CAD build for the part. Positions are in the model's coordinates, mm. A direction names the side the tool comes from. Round coordinates to 2 decimals unless told otherwise and drop trailing zeros. Loops run counter-clockwise (first coordinate to the right, second up) from the corner with the lowest first, then second, coordinate; pieces in that order, holes last. Notation, with made-up numbers: M 57,34.5 L 109,34.5 A20 ccw 109,50.5 Z; hole C 25,-21.75 d4. An arc over 180 degrees is marked long. One line per item, written item: value. Start each with the question number.
from build123d import *

# Parameters (mm, degrees)
SKETCH1_W           = 105
SKETCH1_H           = 70
BOSS_EXTRUDE1_DEPTH = 15
SKETCH3_W           = 98
SKETCH3_H           = 63
CUT_EXTRUDE1_DEPTH  = 12
FILLET1_R           = 6
SKETCH4_R           = 3.5
BOSS_EXTRUDE2_DEPTH = 5
SKETCH5_R           = 1
CUT_EXTRUDE2_DEPTH  = 8
SKETCH6_W           = 3.5
SKETCH6_H           = 18.3
SKETCH6_W_2         = 14
SKETCH6_H_2         = 3.5
SKETCH6_H_3         = 20
CUT_EXTRUDE3_DEPTH  = 6
BOSS_EXTRUDE3_DEPTH = 3
FILLET2_R           = 0.5


with BuildPart() as part:
    # Sketch1 → Boss-Extrude1 (new body)
    with BuildSketch(Plane(origin=(0, 0, 0), x_dir=(1, 0, 0), z_dir=(0, 1, 0))):
        Rectangle(SKETCH1_W, SKETCH1_H)
    extrude(amount=BOSS_EXTRUDE1_DEPTH)

    # Sketch3 → Cut-Extrude1 (cut)
    with BuildSketch(Plane(origin=(0, 15, 0), x_dir=(1, 0, 0), z_dir=(0, 1, 0))):
        Rectangle(SKETCH3_W, SKETCH3_H)
    extrude(amount=-CUT_EXTRUDE1_DEPTH, mode=Mode.SUBTRACT)

    # Fillet1
    fillet1_edges = [part.edges().sort_by_distance(p)[0] for p in [
        (-49, 9, 31.5),
        (-49, 9, -31.5),
        (49, 9, -31.5),
        (49, 9, 31.5),
        (52.5, 7.5, 35),
        (-52.5, 7.5, 35),
        (-52.5, 7.5, -35),
        (52.5, 7.5, -35),
    ]]
    fillet(fillet1_edges, radius=FILLET1_R)

    # Sketch4 → Boss-Extrude2 (add)
    with BuildSketch(Plane(origin=(0, 3, 0), x_dir=(1, 0, 0), z_dir=(0, 1, 0))):
        with Locations(Location((40, -22.5, 0), (0, 0, 270))):
            Circle(SKETCH4_R)
        with Locations(Location((40, 19.2, 0), (0, 0, 270))):
            Circle(SKETCH4_R)
        with Locations(Location((-36.1, -22.5, 0), (0, 0, 270))):
            Circle(SKETCH4_R)
        with Locations(Location((-36.1, 19.2, 0), (0, 0, 270))):
            Circle(SKETCH4_R)
    extrude(amount=BOSS_EXTRUDE2_DEPTH)

    # Sketch5 → Cut-Extrude2 (cut)
    with BuildSketch(Plane(origin=(0, 8, 0), x_dir=(1, 0, 0), z_dir=(0, 1, 0))):
        with Locations(Location((-36.1, 19.2, 0), (0, 0, 270))):
            Circle(SKETCH5_R)
        with Locations(Location((-36.1, -22.5, 0), (0, 0, 270))):
            Circle(SKETCH5_R)
        with Locations(Location((40, -22.5, 0), (0, 0, 270))):
            Circle(SKETCH5_R)
        with Locations(Location((40, 19.06026255, 0), (0, 0, 270))):
            Circle(SKETCH5_R)
    extrude(amount=-CUT_EXTRUDE2_DEPTH, mode=Mode.SUBTRACT)

    # Sketch6 → Cut-Extrude3 (cut)
    with BuildSketch(Plane(origin=(0, 15, 0), x_dir=(1, 0, 0), z_dir=(0, 1, 0))):
        with Locations((50.75, 0.51)):
            Rectangle(SKETCH6_W, SKETCH6_H)
        with Locations((27.76, -33.25)):
            Rectangle(SKETCH6_W_2, SKETCH6_H_2)
        with Locations((-50.75, 0)):
            Rectangle(SKETCH6_W, SKETCH6_H_3)
    extrude(amount=-CUT_EXTRUDE3_DEPTH, mode=Mode.SUBTRACT)

    # Sketch7 → Boss-Extrude3 (add)
    with BuildSketch(Plane(origin=(0, 15, 0), x_dir=(1, 0, 0), z_dir=(0, 1, 0))):
        with BuildLine():
            Line((-44.5, 33), (44.5, 33))
            ThreePointArc((44.5, 33), (48.742640687, 31.242640687), (50.5, 27))
            Line((50.5, 27), (50.5, 9.736559035))
            Line((50.5, 9.736559035), (48.5, 9.736559035))
            Line((48.5, 9.736559035), (48.5, 25))
            ThreePointArc((48.5, 25), (46.742640687, 29.242640687), (42.5, 31))
            Line((42.5, 31), (-42.5, 31))
            ThreePointArc((-42.5, 31), (-46.742640687, 29.242640687), (-48.5, 25))
            Line((-48.5, 25), (-48.5, 10))
            Line((-48.5, 10), (-50.5, 10))
            Line((-50.5, 10), (-50.5, 27))
            ThreePointArc((-50.5, 27), (-48.742640687, 31.242640687), (-44.5, 33))
        make_face()
        with BuildLine():
            Line((-44.5, -33), (20.754470261, -33))
            Line((20.754470261, -33), (20.754470261, -31))
            Line((20.754470261, -31), (-42.5, -31))
            ThreePointArc((-42.5, -31), (-46.742640687, -29.242640687), (-48.5, -25))
            Line((-48.5, -25), (-48.5, -10.02702289))
            Line((-48.5, -10.02702289), (-50.5, -10.02702289))
            Line((-50.5, -10.02702289), (-50.5, -27))
            ThreePointArc((-50.5, -27), (-48.742640687, -31.242640687), (-44.5, -33))
        make_face()
        with BuildLine():
            Line((50.5, -8.739580153), (50.5, -27))
            ThreePointArc((50.5, -27), (48.742640687, -31.242640687), (44.5, -33))
            Line((44.5, -33), (34.809182833, -33))
            Line((34.809182833, -33), (34.809182833, -31))
            Line((34.809182833, -31), (42.5, -31))
            ThreePointArc((42.5, -31), (46.742640687, -29.242640687), (48.5, -25))
            Line((48.5, -25), (48.5, -8.739580153))
            Line((48.5, -8.739580153), (50.5, -8.739580153))
        make_face()
    extrude(amount=BOSS_EXTRUDE3_DEPTH)

    # Fillet2
    fillet2_edges = [part.edges().sort_by_distance(p)[0] for p in [
        (49, 15, 17.119790077),
        (47.242640687, 15, 29.742640687),
        (-49, 15, 17.763511445),
        (-47.242640687, 15, 29.742640687),
        (49, 15, -17.618279517),
        (47.242640687, 15, -29.742640687),
        (-49, 15, -17.75),
        (-47.242640687, 15, -29.742640687),
        (38.904591417, 15, 31.5),
        (-11.12276487, 15, 31.5),
        (0, 15, -31.5),
    ]]
    fillet(fillet2_edges, radius=FILLET2_R - 0.0001)  # a hair under: the kernel refuses the full size


solid = part.part
(1) Flat gauge pins, fed straight in: P1, Ø0.6, axis at y = 17, z = 32, coming from the -X side; P2, Ø7.5, axis at x = -37, z = -20.5, coming from the +Y side; P3, Ø3, axis at y = 12.5, z = 32.5, coming from the +X side; P4, Ø4, axis at x = 28.5, y = 9.5, coming from the +Z side. Where does each tip first touch, or does it go through?
(2) Slice it at A-A, the plane y = 13.25. List the corners of the cut face in (x, z), and give its area (3 significant figures).
(3) Probe L1, parallel to X at y = 3.25, z = 22.5; L2, parallel to X at y = 6.75, z = 24; L3, parallel to Z at x = -6, y = 9.5. List the from-to ranges inside material, lowest first.
(4) Slice it at D-D, the plane z = 3.5. List the corners of the cut face in (x, y).
(5) Which spindle directions (+Z, -Z, +X, -X, +Y, -Y) get a long thin tool onto all of the face, cutting with end or side? Do faces 4 (the flat face through (-50.5, 16, -18)), 5 (the cylindrical face through (-32.63, 5.46, 22.04)), 6 (the flat face through (34.809, 17, 32)), 7 (the flat face through (-49, 17, 10.027)). Say none if no direction does.
(6) Mould opens along X. For faces 1 (the cylindrical face through (-35.26, 4.06, 23.04)), 2 (the flat face through (11, 18, -32)), 3 (the cylindrical face through (48.789, 16.479, 31.196)) say: pulls with the +X half, pulls with the -X half, needs draft (parallel to the pull), parting line crosses it, or undercut.
Check result:
1. P1: stops at x = -48.23
1. P2: stops at y = 8
1. P3: stops at x = 52.16
1. P4: stops at z = 35
2. outline: M -52.5,-29 A6 ccw -46.5,-35 L 46.5,-35 A6 ccw 52.5,-29 L 52.5,-9.66 L 49,-9.66 L 49,-25.5 A6 cw 43,-31.5 L -43,-31.5 A6 cw -49,-25.5 L -49,-10 L -52.5,-10 Z; M -52.5,10 L -49,10 L -49,25.5 A6 cw -43,31.5 L 20.76,31.5 L 20.76,35 L -46.5,35 A6 ccw -52.5,29 Z; M 34.76,31.5 L 43,31.5 A6 cw 49,25.5 L 49,8.64 L 52.5,8.64 L 52.5,29 A6 ccw 46.5,35 L 34.76,35 Z
2. area: 993 mm^2
3. L1: x = -52.5 to -49, -39.6 to -37.1, -35.1 to -32.6, 36.5 to 39, 41 to 43.5, 49 to 52.5
3. L2: x = -52.5 to -49, -39.26 to -32.94, 36.84 to 43.16, 49 to 52.5
3. L3: z = -35 to -31.5, 31.5 to 35
4. outline: M -52.5,0 L 52.5,0 L 52.5,9 L 49,9 L 49,3 L -49,3 L -49,9 L -52.5,9 Z
5. face 4: +Z, -Z, -X, +Y
5. face 5: +Y
5. face 6: +Z, +Y
5. face 7: -X, +Y
6. face 1: undercut
6. face 2: needs draft
6. face 3: pulls with the +X half
